```python
from build123d import *

# Parameters (mm, degrees)
CHAMFER_1_SIZE           = 1
CUT_EXTRUDE_1_DEPTH      = 65
PATTERN_CIRCULAR_1_COUNT = 8


with BuildPart() as part:
    # Sketch 1 → Revolve 1 (revolve)
    with BuildSketch(Plane(origin=(0, 0, 0), x_dir=(0, 0, -1), z_dir=(1, 0, 0)), mode=Mode.PRIVATE) as revolve_1_sk:
        Polygon((0, 46), (0, 65), (56, 65), (56, 46), (126, 46), (126, 32), (123, 32), (123, 34), (45, 34), (45, 46), align=None)
    revolve(revolve_1_sk.sketch.rotate(Axis((0, 0, 0), (0, 0, -1)), 90), axis=Axis((0, 0, 0), (0, 0, -1)))

    # Chamfer 1
    chamfer_1_edges = [part.edges().sort_by_distance(p)[0] for p in [
        (-46, 0, 0),
        (-65, 0, 0),
    ]]
    chamfer(chamfer_1_edges, length=CHAMFER_1_SIZE)

    # Sketch 2 → Cut-Extrude 1 (cut)
    with BuildSketch(Plane(origin=(0, 65, -28), x_dir=(-1, 0, 0), z_dir=(0, 1, 0))):
        Polygon((16, 28), (-16, 28), (-9.198190027, -4), (9.198190027, -4), align=None)
    cut_extrude_1 = extrude(amount=-CUT_EXTRUDE_1_DEPTH, mode=Mode.SUBTRACT)

    # Pattern Circular 1: Cut-Extrude 1 ×8 about axis
    pattern_circular_1_axis = Axis((0, 0, 0), (0, 0, 1))
    for i in range(1, PATTERN_CIRCULAR_1_COUNT):
        add(cut_extrude_1.rotate(pattern_circular_1_axis, i * 360 / PATTERN_CIRCULAR_1_COUNT), mode=Mode.SUBTRACT)


solid = part.part
```
The model under review builds one solid part; all positions refer to its coordinate system, in mm. A direction names the side the tool comes from. Round coordinates to 2 decimals unless told otherwise and drop trailing zeros. Loops run counter-clockwise (first coordinate to the right, second up) from the corner with the lowest first, then second, coordinate; pieces in that order, holes last. Notation, with made-up numbers: (29, 6.5) -> (39, 6.5) arc R20 cw to (39, 35.5) -> close; hole circle Ø3 at (-11.75, 1.25). An arc over 180 degrees is marked (long way). Answer as a JSON object with one key per item and string values. Group by question number.
1) We need section D-D on y = -50. Write out the cut boundary in (x, z).
2) We need section C-C on z = -100. Write out the cut boundary in (x, y).
3) We need section A-A on y = 0. Write out the cut boundary in (x, z), then the cut area to 3 significant figures.
4) For faces 1 (the face through (60, 25, -35)), 2 (the face through (39, 39, -32)), 3 (the face through (-12.551, 53.924, -16.224)), 4 (the face through (53.924, -12.647, -15.776)), list the 3-axis set-ups (+Z, -Z, +X, -X, +Y, -Y) from which the entire face can be reached by the end or side of a thin tool; tool diameter is ignored.
5) For line 1 (Y direction, x = 0, z = -123.9); line 2 (Y direction, x = 0, z = -102); line 3 (Z direction, x = -9.5, y = -37), list the stretches that pass through material, from the lowest coordinate up. Write a range as [from, to].
6) For pin 1 Ø9 at (x, y) = (-53.5, -4) entering from +Z; pin 2 Ø2 at (y, z) = (-7, -97) entering from -X; pin 3 Ø1 at (x, z) = (2.5, -97) entering from -Y; pin 4 Ø20.5 at (x, y) = (16.5, -12.5) entering from +Z, all flat-tipped, find the tip position at first contact; note any pin that passes through.
Result set:
{
 "1": {"outline": "(-41.53, -56) -> (41.53, -56) -> (41.53, -32) -> (36.99, -32) -> (27.37, 0) -> (16, 0) -> (9.2, -32) -> (-9.2, -32) -> (-16, 0) -> (-27.37, 0) -> (-36.99, -32) -> (-41.53, -32) -> close"},
 "2": {"outline": "circle Ø92 at (0, 0); hole circle Ø68 at (0, 0)"},
 "3": {"outline": "(-65, -56) -> (-46, -56) -> (-46, -126) -> (-32, -126) -> (-32, -123) -> (-34, -123) -> (-34, -45) -> (-46, -45) -> (-46, -32) -> (-65, -32) -> close; (32, -126) -> (46, -126) -> (46, -56) -> (65, -56) -> (65, -32) -> (46, -32) -> (46, -45) -> (34, -45) -> (34, -123) -> (32, -123) -> close", "area": "2,870 mm²"},
 "4": {"face 1": "+Z, -Z", "face 2": "+Z", "face 3": "+Z, +Y, -Y", "face 4": "+Z, +X, -X"},
 "5": {"line 1": "[-46, -32], [32, 46]", "line 2": "[-46, -34], [34, 46]", "line 3": "[-126, -45]"},
 "6": {"pin 1": "z = -32", "pin 2": "x = -45.61", "pin 3": "y = -45.96", "pin 4": "through"}
}
